from build123d import *

# Parameters (mm, degrees)
SKETCH2_W           = 60
SKETCH2_H           = 42.3
BOSS_EXTRUDE1_DEPTH = 13
SKETCH3_R           = 4.015
CUT_EXTRUDE1_DEPTH  = 10
CUT_EXTRUDE2_DEPTH  = 3
SKETCH5_R           = 3.75
CUT_EXTRUDE3_DEPTH  = 41.498999822
CUT_EXTRUDE4_DEPTH  = 3


with BuildPart() as part:
    # Sketch2 → Boss-Extrude1 (new body)
    with BuildSketch(Plane.XY):
        with Locations((1.553418124, -2.185612083)):
            Rectangle(SKETCH2_W, SKETCH2_H)
    extrude(amount=BOSS_EXTRUDE1_DEPTH)

    # Sketch3 → Cut-Extrude1 (cut)
    with BuildSketch(Plane.XY.offset(13)):
        with Locations((22.703418124, -2.185612083)):
            Circle(SKETCH3_R)
        with Locations(Location((-19.596581876, -2.185612083, 0), (0, 0, 180))):
            Circle(SKETCH3_R)
    extrude(amount=-CUT_EXTRUDE1_DEPTH, mode=Mode.SUBTRACT)

    # Sketch4 → Cut-Extrude2 (cut)
    with BuildSketch(Plane.XY.offset(13)):
        Polygon((9.076292132, -2.185612083), (5.314855128, 4.329387917), (-2.20801888, 4.329387917), (-5.969455884, -2.185612083), (-2.20801888, -8.700612083), (5.314855128, -8.700612083), align=None)
    extrude(amount=-CUT_EXTRUDE2_DEPTH, mode=Mode.SUBTRACT)

    # Sketch5 → Cut-Extrude3 (cut, through all)
    with BuildSketch(Plane.XY.offset(10)):
        with Locations((1.553418124, -2.185612083)):
            Circle(SKETCH5_R)
    extrude(amount=-CUT_EXTRUDE3_DEPTH, mode=Mode.SUBTRACT)

    # Sketch6 → Cut-Extrude4 (cut)
    with BuildSketch(Plane(origin=(0, 0, 0), x_dir=(-1, 0, 0), z_dir=(0, 0, -1))):
        Polygon((5.969455884, -2.185612083), (2.20801888, 4.329387917), (-5.314855128, 4.329387917), (-9.076292132, -2.185612083), (-5.314855128, -8.700612083), (2.20801888, -8.700612083), align=None)
    extrude(amount=-CUT_EXTRUDE4_DEPTH, mode=Mode.SUBTRACT)


solid = part.part
Read the model definition and answer for the solid it produces. Units are mm, in the model's axes. A direction names the side the tool comes from. Give positions to 0.01 mm unless a question says otherwise; leave off trailing zeros. Loops run counter-clockwise (first coordinate to the right, second up) from the corner with the lowest first, then second, coordinate; pieces in that order, holes last. Notation, with made-up numbers: (55.25, 54) -> (84.25, 54) arc R24 ccw to (84.25, 87) -> close; hole circle Ø6 at (43.5, 33). An arc over 180 degrees is marked (long way). Use a Markdown table: item, result.
Q1. Find the intervals of material crossed by line 1 along Y through (x, z) = (-21, 9.25); line 2 along Y through (x, z) = (5, 11.5); line 3 along X through (y, z) = (0.5, 4.5), in increasing order.
Solved:
| item | result |
|---|---|
| line 1 | y = -23.34 to -5.95, 1.58 to 18.96 |
| line 2 | y = -23.34 to -8.7, 4.33 to 18.96 |
| line 3 | x = -28.45 to -22.58, -16.61 to -1.06, 4.17 to 19.72, 25.69 to 31.55 |
Q2. A tool of negligible diameter and unlimited length cuts with its end or side. For faces 1 (the face through (23, -2, 3)), 2 (the face through (-6, 3, 13)), 3 (the face through (2, -8.701, 1)), from which of +Z, -Z, +X, -X, +Y, -Y can it reach the whole face along a straight path? Write none if from no direction.
Solved:
| item | result |
|---|---|
| face 1 | +Z |
| face 2 | +Z, +X, -X, +Y, -Y |
| face 3 | -Z |
Q3. Section D-D, the plane z = 11.25 is taken. Determine the outline of the cut face in (x, y) (3 decimals), then the cut area to 3 significant figures.
Solved:
| item | result |
|---|---|
| outline | (-28.447, -23.336) -> (31.553, -23.336) -> (31.553, 18.964) -> (-28.447, 18.964) -> close; hole circle Ø8.03 at (-19.597, -2.186); hole (-5.969, -2.186) -> (-2.208, -8.701) -> (5.315, -8.701) -> (9.076, -2.186) -> (5.315, 4.329) -> (-2.208, 4.329) -> close; hole circle Ø8.03 at (22.703, -2.186) |
| area | 2,290 mm^2 |
Q4. Each of these flat-tipped pins is pushed along its axis until it touches: pin 1 (10 mm diameter, centred on x = 1.55, y = -2.19, fed in from +Z); pin 2 (5 mm diameter, centred on x = 14, y = 13, fed in from -Z); pin 3 (5 mm diameter, centred on x = 24, y = -2.5, fed in from +Z). Where does it stop, or does it pass through?
Solved:
| item | result |
|---|---|
| pin 1 | stops at z = 10 |
| pin 2 | stops at z = 0 |
| pin 3 | stops at z = 3 |
Q5. Section C-C, the plane y = -4 is taken. Determine the outline of the cut face in (x, z), then the cut area to 3 significant figures.
Solved:
| item | result |
|---|---|
| outline | (-28.45, 0) -> (-4.92, 0) -> (-4.92, 3) -> (-1.73, 3) -> (-1.73, 10) -> (-4.92, 10) -> (-4.92, 13) -> (-16.01, 13) -> (-16.01, 3) -> (-23.18, 3) -> (-23.18, 13) -> (-28.45, 13) -> close; (4.84, 3) -> (8.03, 3) -> (8.03, 0) -> (31.55, 0) -> (31.55, 13) -> (26.29, 13) -> (26.29, 3) -> (19.12, 3) -> (19.12, 13) -> (8.03, 13) -> (8.03, 10) -> (4.84, 10) -> close |
| area | 513 mm^2 |
Q6. Section B-B, the plane z = 5.75 is taken. Determine the outline of the cut face in (x, y) (3 decimals).
Solved:
| item | result |
|---|---|
| outline | (-28.447, -23.336) -> (31.553, -23.336) -> (31.553, 18.964) -> (-28.447, 18.964) -> close; hole circle Ø8.03 at (-19.597, -2.186); hole circle Ø7.5 at (1.553, -2.186); hole circle Ø8.03 at (22.703, -2.186) |
Q7. Section A-A, the plane x = -0.5 is taken. Determine the outline of the cut face in (y, z), then the cut area to 3 significant figures.
Solved:
| item | result |
|---|---|
| outline | (-23.34, 0) -> (-8.7, 0) -> (-8.7, 3) -> (-5.32, 3) -> (-5.32, 10) -> (-8.7, 10) -> (-8.7, 13) -> (-23.34, 13) -> close; (0.95, 3) -> (4.33, 3) -> (4.33, 0) -> (18.96, 0) -> (18.96, 13) -> (4.33, 13) -> (4.33, 10) -> (0.95, 10) -> close |
| area | 428 mm^2 |
Q8. Determine the mould class of faces 4 (the face through (7.17, 1.12, 1.48)), 5 (the face through (31.553, -2, 6)) for opening direction Y: pulls with the +Y half, pulls with the -Y half, needs draft (parallel to the pull), parting line crosses it, or undercut.
Solved:
| item | result |
|---|---|
| face 4 | undercut |
| face 5 | needs draft |
